For this review, take the finished solid that the model builds, in its own axes (mm). Face numbers are marked on the shaded views. A direction names the side the tool comes from. Coordinates: 2 decimals unless noted, no trailing zeros. Order: outer loops, then holes, each group sorted by start corner. A loop starts at its lowest first (then second) coordinate and runs counter-clockwise, first axis right, second up. Notation, with made-up numbers: (56.25, 73) -> (74.25, 73) arc R28 ccw to (74.25, 101) -> close; hole circle Ø9 at (36, 48). An arc over 180 degrees is marked (long way). Return JSON: item names as keys, results as strings. Group by question number.
Item 1: Insertion check: pin 1 (2.5 mm diameter, centred on x = -0.5, z = -23.5, fed in from -Y); pin 2 (2.5 mm diameter, centred on x = -1, z = -23, fed in from +Y); pin 3 (5 mm diameter, centred on x = 10.5, y = -16, fed in from +Z). Each pin has a flat end and moves straight along its axis. Give the tip position at first contact, or say it passes through.
Item 2: For line 1 along X through (y, z) = (0, -20.5); line 2 along Y through (x, z) = (0, -13); line 3 along Z through (x, y) = (15.5, -14), list the stretches that pass through material, from the lowest coordinate up.
Item 3: Machinability: for the marked faces 1, 2 and 3, which of the approach directions +Z, -Z, +X, -X, +Y, -Y give a long, thin tool a straight path to every point of the face, cutting with its end or side? Answer none if there is none.
Item 4: Take a section at A-A (z = 81). Write out the cut boundary in (x, y), then the cut area to 3 significant figures.
```python
from build123d import *

# Parameters (mm, degrees)
EXTRUDE_1_DEPTH     = 200
SKETCH_2_R          = 15
EXTRUDE_2_DEPTH     = 3
SKETCH_3_R          = 13
EXTRUDE_3_DEPTH     = 14.5
SKETCH_4_R          = 8
EXTRUDE_4_DEPTH     = 7.5
SKETCH_5_R          = 10
EXTRUDE_5_DEPTH     = 16
CUT_EXTRUDE_START   = -5
CUT_EXTRUDE_1_DEPTH = 5
M10X1_25_1_D        = 8.8
M10X1_25_1_DEPTH    = 15
M10X1_25_1_TIP      = 2.643786724


with BuildPart() as part:
    # 스케치1 → 보스-돌출1 (new body)
    with BuildSketch(Plane.XY):
        Polygon((-21, 16), (-16, 21), (16, 21), (21, 16), (21, -16), (16, -21), (-16, -21), (-21, -16), align=None)
    extrude(amount=EXTRUDE_1_DEPTH)

    # 스케치2 → 보스-돌출2 (add)
    with BuildSketch(Plane.XY):
        Circle(SKETCH_2_R)
    extrude(amount=-EXTRUDE_2_DEPTH)

    # 스케치3 → 보스-돌출3 (add)
    with BuildSketch(Plane(origin=(0, 0, -3), x_dir=(-1, 0, 0), z_dir=(0, 0, -1))):
        with Locations(Location((0, 0, 0), (0, 0, 180))):
            Circle(SKETCH_3_R)
    extrude(amount=EXTRUDE_3_DEPTH)

    # 스케치4 → 보스-돌출4 (add)
    with BuildSketch(Plane(origin=(0, 0, -17.5), x_dir=(-1, 0, 0), z_dir=(0, 0, -1))):
        Circle(SKETCH_4_R)
    extrude(amount=EXTRUDE_4_DEPTH)

    # 스케치5 → 보스-돌출5 (add)
    with BuildSketch(Plane.XY.offset(200)):
        Circle(SKETCH_5_R)
    extrude(amount=EXTRUDE_5_DEPTH)

    # 스케치6 → 컷-돌출1 (cut)
    with BuildSketch(Plane(origin=(0, 0, -25), x_dir=(-1, 0, 0), z_dir=(0, 0, -1)).offset(CUT_EXTRUDE_START)):
        with BuildLine():
            Line((-5.291502622, 6), (5.291502622, 6))
            ThreePointArc((5.291502622, 6), (0, 8), (-5.291502622, 6))
        make_face()
        with BuildLine():
            Line((-5.291502622, -6), (5.291502622, -6))
            ThreePointArc((5.291502622, -6), (0, -8), (-5.291502622, -6))
        make_face()
    extrude(amount=CUT_EXTRUDE_1_DEPTH, mode=Mode.SUBTRACT)

    # M10x1.25 탭을 위한 탭 드릴1
    with Locations(Plane(origin=(0, 0, -25), x_dir=(-1, 0, 0), z_dir=(0, 0, -1))):
        with Locations((0, 0)):
            Hole(M10X1_25_1_D / 2, depth=M10X1_25_1_DEPTH)
            with Locations((0, 0, -(M10X1_25_1_DEPTH + M10X1_25_1_TIP / 2))):  # 118° drill point
                Cone(0, M10X1_25_1_D / 2, M10X1_25_1_TIP, mode=Mode.SUBTRACT)


solid = part.part
```
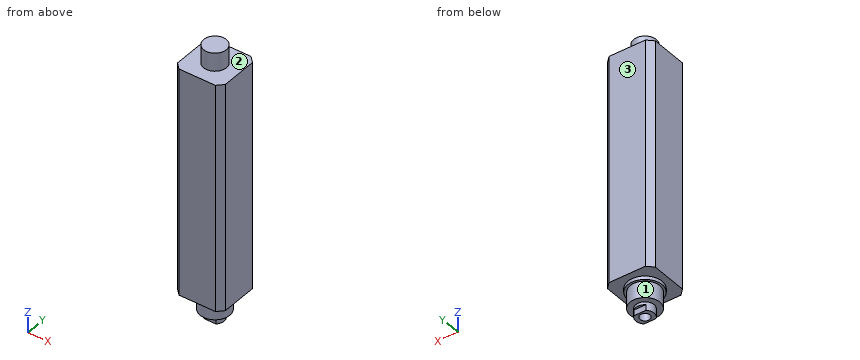
Findings below:
{
 "1": {"pin 1": "stops at y = -6", "pin 2": "stops at y = 6", "pin 3": "stops at z = 200"},
 "2": {"line 1": "x = -8 to -4.4, 4.4 to 8", "line 2": "y = -13 to -4.4, 4.4 to 13", "line 3": "z = 0 to 200"},
 "3": {"face 1": "-Z", "face 2": "+Z", "face 3": "+Z, -Z, +X, -X, +Y"},
 "4": {"outline": "(-21, -16) -> (-16, -21) -> (16, -21) -> (21, -16) -> (21, 16) -> (16, 21) -> (-16, 21) -> (-21, 16) -> close", "area": "1,710 mm2"}
}
